Check sheet for the modelled part. Datum: model origin and axes. Units: mm. Face numbers are marked on the shaded views. A direction names the side the tool comes from. Give positions to 0.01 mm unless a question says otherwise; leave off trailing zeros. Order: outer loops, then holes, each group sorted by start corner. A loop starts at its lowest first (then second) coordinate and runs counter-clockwise, first axis right, second up.
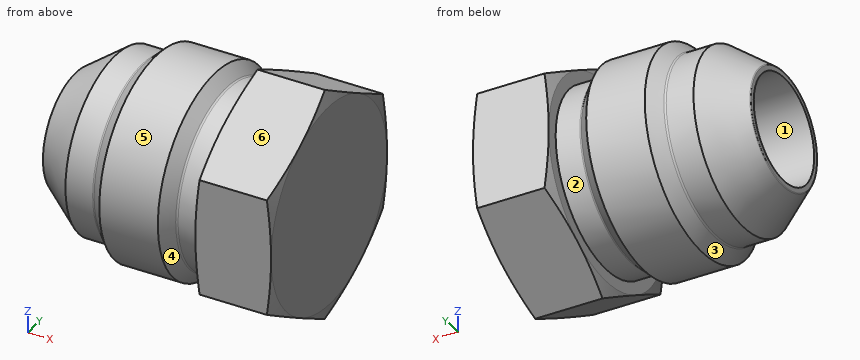
Autodesk Inventor part; units mm, degrees
ref_plane "Work Plane3" through (11.9062, 0, 0) normal (-1, 0, 0) x (0, 0, 1)
ref_plane "YZ Plane" through (0, 0, 0) normal (1, 0, 0) x (0, 1, 0)
ref_plane "XZ Plane" through (0, 0, 0) normal (0, 1, 0) x (-1, 0, 0)
sketch "Sketch4" plane through (0, 0, 0) normal (0, 0, 1) x (1, 0, 0)
  line L0 (0, 0) -> (0, 5.4102)
  line L1 (0.0506, 5.5116) -> (3.7586, 8.3058)
  line L2 (3.7586, 8.3058) -> (6.321, 8.3058)
  line L3 (6.5006, 8.3802) -> (7.6454, 9.525)
  line L4 (7.6454, 9.525) -> (13.1572, 9.525)
  line L5 (13.1572, 9.525) -> (14.2258, 8.4564)
  line L6 (14.4054, 8.382) -> (16.6878, 8.382)
  line L7 (16.6878, 8.382) -> (16.6878, 0)
  line L8 (16.6878, 0) -> (0, 0)
  arc A0 (0.0506, 5.5116) -> (0, 5.4102) centre (0.127, 5.4102) ccw
  arc A1 (6.321, 8.3058) -> (6.5006, 8.3802) centre (6.321, 8.5598) ccw
  arc A2 (14.2258, 8.4564) -> (14.4054, 8.382) centre (14.4054, 8.636) ccw
  point P0 (6.4262, 8.3058)
  point P1 (14.3002, 8.382)
  dimension "d26" = 45
  dimension "d28" = 16.6878
  dimension "d29" = 0.127
  dimension "d30" = 5.4102
  dimension "d31" = 37
  dimension "d32" = 6.4262
  dimension "d33" = 8.3058
  dimension "d34" = 0.254
  dimension "d35" = 8.382
  dimension "d36" = 9.525
  dimension "d37" = 45
  dimension "d39" = 2.3876
revolve "Revolution3" add sketch "Sketch4" angle 360 about axis through (16.6878, 0, 0) along (-1, 0, 0)
ref_plane "Work Plane3" through (11.9062, 0, 0) normal (-1, 0, 0) x (0, 0, 1)
sketch "Sketch5" plane through (16.6878, 8.382, 0) normal (-1, 0, 0) x (0, -1, 0)
  line L0 (-1.143, 5.4993) -> (8.382, 10.9985)
  line L1 (8.382, 10.9985) -> (17.907, 5.4993)
  line L2 (17.907, 5.4993) -> (17.907, -5.4993)
  line L3 (17.907, -5.4993) -> (8.382, -10.9985)
  line L4 (8.382, -10.9985) -> (-1.143, -5.4993)
  line L5 (-1.143, -5.4993) -> (-1.143, 5.4993)
  circle A0 centre (8.382, 0) radius 10.9985 construction
  dimension "d42" = 21.9971
  dimension "d41" = 19.05
extrude "Extrusion2" add sketch "Sketch5" against normal blind 7.1247
sketch "Sketch7" plane through (0, 0, 0) normal (-1, 0, 0) x (0, 0, 1)
  circle A0 centre (0, 0) radius 5.4102
hole "Hole1" at (0, 0, 0) direction (1, 0, 0) diameter 9.9314 depth 15.875 tip angle 118
thread "Thread3"
sketch "Sketch8" plane through (0, 0, 0) normal (0, 1, 0) x (-1, 0, 0)
  line L0 (-14.4054, 8.382) -> (-16.6878, 8.382) construction
  line L1 (-16.6878, 5.4993) -> (-16.6878, 10.9985) construction
  line L2 (-16.6878, 5.4993) -> (-16.6878, 10.9985) construction
  line L3 (-16.6878, 10.9985) -> (-23.8125, 10.9985) construction
  line L4 (-16.6878, 5.4993) -> (-23.8125, 5.4993) construction
  line L5 (-17.0826, 10.9985) -> (-16.6878, 9.525)
  line L6 (-17.0826, 10.9985) -> (-16.6878, 10.9985)
  line L7 (-16.6878, 9.525) -> (-16.6878, 10.9985)
  line L8 (-20.2502, 10.9985) -> (-20.2502, 5.4993)
  line L9 (-23.4177, 10.9985) -> (-23.8125, 9.525)
  line L10 (-23.4177, 10.9985) -> (-23.8125, 10.9985)
  line L11 (-23.8125, 9.525) -> (-23.8125, 10.9985)
  line L12 (8.8106, 0) -> (-52.8638, 0)
  line L13 (-23.8125, 5.4993) -> (-23.8125, 10.9985)
  point P0 (0, 0)
  point P1 (-23.8125, 10.9985)
  dimension "d62" = 9.525
  dimension "d64" = 15
revolve "Revolution5" cut sketch "Sketch8" angle 360 about axis through (-10, 0, 0) along (1, 0, 0)
equation "\"d28\" = MS33656_J"
equation "\"d30\" = 0.5 * MS33656_D"
equation "\"d33\" = 0.5 * MS33656_C"
equation "\"d35\" = 0.5 * MS33656_F"
equation "\"d36\" = 0.5 * AN806_T"
equation "\"d41\" = AN806_C"
equation "\"d44\" = AN806_B - MS33656_J"
equation "\"d53\" = MS33656_A"
equation "\"d58\" = AN806_A"
equation "\"AN806_T\" = 19.05"
equation "\"AN806_C\" = 19.05"
equation "\"AN806_B\" = 23.8125"
equation "\"MS33656_A\" = 9.9314"
equation "\"MS33656_D\" = 10.8204"
equation "\"MS33656_B\" = 6.4262"
equation "\"MS33656_C\" = 16.6116"
equation "\"MS33656_F\" = 16.764"
equation "\"MS33656_J\" = 16.6878"
equation "\"MS33656_Q\" = 2.3876"
equation "\"d79\" = -0.5 * AN806_B"
equation "\"Tube_OD\" = 12.7"
equation "\"AN806_A\" = 15.875"
properties part number "AN815-8D" material "Aluminum 2014-T6"
(1) Release check for a two-part mould opening along X. For the marked faces 1, 2 and 3 record: released by +X, released by -X, zero draft, split by the parting line, or undercut.
Response values:
face 1: zero draft
face 2: undercut
face 3: released by -X
(2) Cross-section at C-C on x = 11.75. Enter the section's corners in (y, z) (3 decimals), then the cut area to 3 significant figures.
Response values:
outline: circle Ø19.05 at (0, 0); hole circle Ø9.931 at (0, 0)
area: 208 mm2
(3) Material ranges on L1, parallel to Z at x = 4, y = 0; L2, parallel to Y at x = 11, z = 0 (3 decimals), recorded low to high.
Response values:
L1: z = -8.31 to -4.97, 4.97 to 8.31
L2: y = -9.525 to -4.966, 4.966 to 9.525
(4) Cross-section at B-B on x = 19.75. Enter the section's corners in (y, z) (1 decimal).
Response values:
outline: (-9.5, -5.5) - (0, -11) - (9.5, -5.5) - (9.5, 5.5) - (0, 11) - (-9.5, 5.5) - close
(5) Gauge pin test, flat ends, axial feed: pin 1 Ø10 at (x, z) = (18.5, -6.5) entering from +Y (3 decimals); pin 2 Ø2 at (x, z) = (12.5, 5.5) entering from +Y (3 decimals); pin 3 Ø10 at (x, y) = (4, 5.5) entering from -Z; pin 4 Ø3 at (x, y) = (4, -6) entering from -Z. Record the tip position at first contact, or that the pin passes through.
Response values:
pin 1: stops at y = 9.525
pin 2: stops at y = 8.395
pin 3: stops at z = -9.3
pin 4: stops at z = -6.98
(6) Set-up check for the marked faces 4, 5 and 6: record each of +Z, -Z, +X, -X, +Y, -Y from which the full face is reachable in a straight line by a thin tool's end or side.
Response values:
face 4: none
face 5: -X
face 6: +Z, +X, -X, -Y
(7) Cross-section at A-A on x = 5.25. Enter the section's corners in (y, z).
Response values:
outline: circle Ø16.61 at (0, 0); hole circle Ø9.93 at (0, 0)
